from build123d import *

# Parameters (mm, degrees)
SKETCH1_W           = 50
SKETCH1_H           = 30
SKETCH1_R           = 2
BOSS_EXTRUDE2_DEPTH = 15
SKETCH1_3_W         = 20
SKETCH1_3_H         = 30
SKETCH1_3_R         = 2
BOSS_EXTRUDE3_DEPTH = 15
FILLET1_R           = 5
SKETCH5_W           = 8
SKETCH5_H           = 70
CUT_EXTRUDE1_DEPTH  = 5


with BuildPart() as part:
    # Sketch1 → Boss-Extrude2 (new body)
    with BuildSketch(Plane(origin=(0, 0, 0), x_dir=(1, 0, 0), z_dir=(0, 1, 0))):
        Rectangle(SKETCH1_W, SKETCH1_H)
        with Locations(Location((-15, 9, 0), (0, 0, 270))):
            Circle(SKETCH1_R, mode=Mode.SUBTRACT)
        with Locations(Location((15, 9, 0), (0, 0, 270))):
            Circle(SKETCH1_R, mode=Mode.SUBTRACT)
        with Locations(Location((15, -9, 0), (0, 0, 270))):
            Circle(SKETCH1_R, mode=Mode.SUBTRACT)
        with Locations(Location((-15, -9, 0), (0, 0, 270))):
            Circle(SKETCH1_R, mode=Mode.SUBTRACT)
    extrude(amount=-BOSS_EXTRUDE2_DEPTH)

    # Sketch1<3> → Boss-Extrude3 (add)
    with BuildSketch(Plane(origin=(0, 0, 0), x_dir=(1, 0, 0), z_dir=(0, 1, 0))):
        with Locations((0, -30)):
            Rectangle(SKETCH1_3_W, SKETCH1_3_H)
        with Locations(Location((0, -35, 0), (0, 0, 270))):
            Circle(SKETCH1_3_R, mode=Mode.SUBTRACT)
        with Locations(Location((0, -20, 0), (0, 0, 270))):
            Circle(SKETCH1_3_R, mode=Mode.SUBTRACT)
    extrude(amount=-BOSS_EXTRUDE3_DEPTH)

    # Fillet1
    fillet1_edges = [part.edges().sort_by_distance(p)[0] for p in [
        (-10, -7.5, 15),
        (10, -7.5, 15),
    ]]
    fillet(fillet1_edges, radius=FILLET1_R)

    # Sketch5 → Cut-Extrude1 (cut)
    with BuildSketch(Plane(origin=(0, 0, 0), x_dir=(1, 0, 0), z_dir=(0, 1, 0))):
        with Locations((0, -13.137566138)):
            Rectangle(SKETCH5_W, SKETCH5_H)
    extrude(amount=-CUT_EXTRUDE1_DEPTH, mode=Mode.SUBTRACT)


solid = part.part
The model under review builds one solid part; all positions refer to its coordinate system, in mm. A direction names the side the tool comes from. Coordinates: 2 decimals unless noted, no trailing zeros. Write each loop counter-clockwise with the first axis right and the second up, starting at its lowest first coordinate (ties: lowest second). Pieces come first, ordered by that corner, then holes. Notation, with made-up numbers: (11.5, 82.5) - (28.5, 82.5) arc R7 ccw to (28.5, 94.5) - close; hole circle Ø11 at (83, -22). An arc over 180 degrees is marked (long way). Answer as a JSON object with one key per item and string values. Group by question number.
1. Add section B-B (x = 0). Give the boundary of the cut face in (y, z).
2. Clearance check with flat-ended pins moving along their axes: pin 1 Ø1 at (y, z) = (-11, 37) entering from +X; pin 2 Ø1.5 at (x, z) = (6.5, -1) entering from +Y; pin 3 Ø8 at (x, y) = (19.5, -7.5) entering from +Z; pin 4 Ø2.5 at (x, z) = (-1, 8) entering from +Y. State where each tip first meets the part, or that it passes through.
3. Add section C-C (y = -7). Give the boundary of the cut face in (x, z).
4. To check wall thickness, follow probe 1 along X at (y, z) = (-5.5, -9); probe 2 along X at (y, z) = (-3.5, 9); probe 3 along Z at (x, y) = (-14.5, -1). State the ranges of each line that lie inside material, in increasing order.
5. Add section A-A (z = 9). Give the boundary of the cut face in (x, y).
6. Add section D-D (z = 24). Give the boundary of the cut face in (x, y), plus the area to 3 significant figures.
7. Machinability: for faces 5 (the face through (-4, -2, 15)), 6 (the face through (12, 0, 8)), 7 (the face through (0, -15, 8)), 8 (the face through (20, -7, 15)), 9 (the face through (-10, -7, 33)), which of the approach directions +Z, -Z, +X, -X, +Y, -Y give a long, thin tool a straight path to every point of the face, cutting with its end or side? Answer none if there is none.
8. Mouldability with a two-part tool opening along X and no side actions: class faces 1 (the face through (25, -7, 0)), 2 (the face through (-13, -7, -9)), 3 (the face through (-25, -7, 0)), 4 (the face through (-20, -7, 15)) as pulls with the +X half, pulls with the -X half, needs draft (parallel to the pull), parting line crosses it, or undercut.
Findings:
{
 "1": {"outline": "(-15, -15) - (-5, -15) - (-5, 18) - (-15, 18) - close; (-15, 22) - (-5, 22) - (-5, 33) - (-15, 33) - close; (-15, 37) - (-5, 37) - (-5, 45) - (-15, 45) - close"},
 "2": {"pin 1": "x = 10", "pin 2": "y = 0", "pin 3": "z = 15", "pin 4": "y = -5"},
 "3": {"outline": "(-25, -15) - (25, -15) - (25, 15) - (15, 15) arc R5 cw to (10, 20) - (10, 45) - (-10, 45) - (-10, 20) arc R5 cw to (-15, 15) - (-25, 15) - close; hole circle Ø4 at (-15, -9); hole circle Ø4 at (-15, 9); hole circle Ø4 at (0, 20); hole circle Ø4 at (0, 35); hole circle Ø4 at (15, -9); hole circle Ø4 at (15, 9)"},
 "4": {"probe 1": "-25 to -17, -13 to 13, 17 to 25", "probe 2": "-25 to -17, -13 to -4, 4 to 13, 17 to 25", "probe 3": "-15 to -10.94, -7.06 to 7.06, 10.94 to 15.03"},
 "5": {"outline": "(-25, -15) - (-17, -15) - (-17, 0) - (-25, 0) - close; (-13, -15) - (13, -15) - (13, 0) - (4, 0) - (4, -5) - (-4, -5) - (-4, 0) - (-13, 0) - close; (17, -15) - (25, -15) - (25, 0) - (17, 0) - close"},
 "6": {"outline": "(-10, -15) - (10, -15) - (10, 0) - (4, 0) - (4, -5) - (-4, -5) - (-4, 0) - (-10, 0) - close", "area": "260 mm²"},
 "7": {"face 5": "+Z, -Z, +Y", "face 6": "+Z, -Z, +X, -X, +Y", "face 7": "+Z, -Z, +X, -X, -Y", "face 8": "+Z, +X, +Y, -Y", "face 9": "+Z, -X, +Y, -Y"},
 "8": {"face 1": "pulls with the +X half", "face 2": "undercut", "face 3": "pulls with the -X half", "face 4": "needs draft"}
}
